Geometry: see drawing. Coordinates: mm, zero at the bounding-box minimum. A direction names the side the tool comes from. Coordinates: 2 decimals unless noted, no trailing zeros. Loops run counter-clockwise (first coordinate to the right, second up) from the corner with the lowest first, then second, coordinate; pieces in that order, holes last.
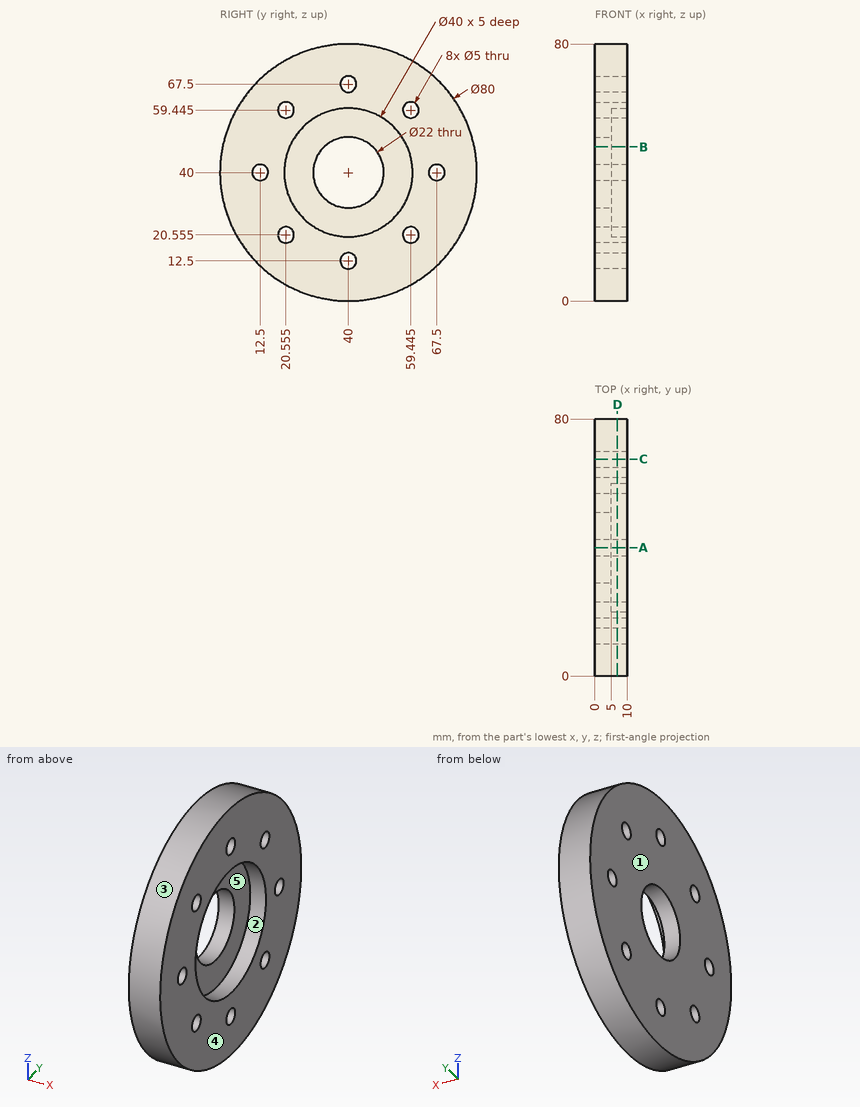
Item 1: Section query D-D (x = 7). Count the separate pieces of the cut face and the enclosed holes in it, then the cut area to 3 significant figures.
Result:
separate pieces: 1
enclosed holes: 9
area: 3,610 mm2
Item 2: Line query: L1, parallel to Y at x = 2.5, z = 40; L2, parallel to Y at x = 3.5, z = 61 (1 decimal); L3, parallel to X at y = 51, z = 29. Output: solid intervals per line, ascending.
Result:
L1: y = 0 to 10, 15 to 29, 51 to 65, 70 to 80
L2: y = 6 to 18.6, 22.5 to 57.5, 61.4 to 74
L3: x = 0 to 5
Item 3: Section query B-B (z = 48). Output: boundary loops of the cut face in (x, y).
Result:
outline: (0, 0.81) - (10, 0.81) - (10, 21.67) - (5, 21.67) - (5, 32.45) - (0, 32.45) - close; (0, 47.55) - (5, 47.55) - (5, 58.33) - (10, 58.33) - (10, 79.19) - (0, 79.19) - close
Item 4: Contact query for flat-ended pins moving along their axis: P1, Ø6, axis at x = 4, z = 62.5, coming from the +Y side (1 decimal); P2, Ø1, axis at x = 7.5, y = 15.5, coming from the +Z side; P3, Ø4, axis at x = 4.5, y = 66.5, coming from the -Z side. Output: stop coordinate, or through.
Result:
P1: stops at y = 74.9
P2: stops at z = 72
P3: stops at z = 8.38
Item 5: Section query A-A (y = 40). Output: boundary loops of the cut face in (x, z).
Result:
outline: (0, 0) - (10, 0) - (10, 10) - (0, 10) - close; (0, 15) - (10, 15) - (10, 20) - (5, 20) - (5, 29) - (0, 29) - close; (0, 51) - (5, 51) - (5, 60) - (10, 60) - (10, 65) - (0, 65) - close; (0, 70) - (10, 70) - (10, 80) - (0, 80) - close
Item 6: Reachability of the marked faces 1 and 2 from +Z, -Z, +X, -X, +Y, -Y: full face, straight path, thin tool, end or side. Return the list, or none.
Result:
face 1: +Z, -Z, -X, +Y, -Y
face 2: +X
Item 7: Section query C-C (y = 67.5). Output: boundary loops of the cut face in (x, z), then the cut area to 3 significant figures.
Result:
outline: (0, 10.95) - (10, 10.95) - (10, 37.5) - (0, 37.5) - close; (0, 42.5) - (10, 42.5) - (10, 69.05) - (0, 69.05) - close
area: 531 mm2
Item 8: Mould query, pull axis Z, two halves, no side actions, for the marked faces 3, 4 and 5. Classes: +Z half, -Z half, draft (parallel to the pull), parting line (faces both ways), or undercut.
Result:
face 3: parting line
face 4: draft
face 5: undercut
